The listing builds one solid part. Answer for the finished solid, in the listing's coordinates (mm). A direction names the side the tool comes from. Coordinates: 2 decimals unless noted, no trailing zeros. Write each loop counter-clockwise with the first axis right and the second up, starting at its lowest first coordinate (ties: lowest second). Pieces come first, ordered by that corner, then holes.
Autodesk Inventor part; units mm, degrees
ref_plane "YZ Plane" through (0, 0, 0) normal (1, 0, 0) x (0, 1, 0)
ref_plane "XZ Plane" through (0, 0, 0) normal (0, 1, 0) x (-1, 0, 0)
ref_plane "XY Plane" through (0, 0, 0) normal (0, 0, 1) x (1, 0, 0)
sketch "Sketch1" plane through (0, 0, 0) normal (0, 1, 0) x (-1, 0, 0)
  line L0 (0, 0) -> (8.89, 0)
  line L1 (8.89, 0) -> (8.89, -16.002)
  line L2 (8.89, -16.002) -> (0, -16.002)
  line L3 (0, -16.002) -> (0, 0)
  dimension "d0" = 8.89
  dimension "d1" = 16.002
extrude "Extrusion1" add sketch "Sketch1" along normal blind 2.54
sketch "Sketch5" plane through (0, 2.54, 0) normal (0, 1, 0) x (1, 0, 0)
  line L0 (-8.89, 0) -> (0, 0)
  line L1 (0, 0) -> (0, 16.002)
  line L2 (0, 16.002) -> (-8.89, 16.002)
  line L3 (-8.89, 16.002) -> (-8.89, 0)
  line L4 (0, 0) -> (-8.89, 0)
  line L5 (-5.7785, 0) -> (-6.6294, 0.9271)
  line L6 (-6.6294, 0.9271) -> (-6.6294, 1.6764)
  line L7 (-6.6294, 1.6764) -> (-2.2606, 1.6764)
  line L8 (-2.2606, 1.6764) -> (-2.2606, 0.9271)
  line L9 (-2.2606, 0.9271) -> (-3.1115, 0)
  line L10 (-8.89, 0) -> (-8.89, 16.002)
  line L11 (-8.89, 3.81) -> (0, 3.81)
  point P0 (-4.445, 1.6764)
  point P1 (-4.445, 3.81)
  dimension "d19" = 2.667
  dimension "d20" = 4.3688
  dimension "d21" = 0.9271
  dimension "d23" = 1.6764
  dimension "d24" = 3.81
extrude "Extrusion4" add sketch "Sketch5" along normal blind 3.175 contours L3 L11 L1 L0 L9 L8 L7 L6 L5
sketch "Sketch6" plane through (0, 2.54, 0) normal (0, 1, 0) x (1, 0, 0)
  line L0 (-3.1115, 0) -> (-2.2606, 0.9271)
  line L1 (-2.2606, 0.9271) -> (-2.2606, 1.6764)
  line L2 (-2.2606, 1.6764) -> (-6.6294, 1.6764)
  line L3 (-6.6294, 1.6764) -> (-6.6294, 0.9271)
  line L4 (-6.6294, 0.9271) -> (-5.7785, 0)
  line L5 (-5.7785, 0) -> (-3.1115, 0)
  point P0 (0, 0)
extrude "Extrusion5" cut sketch "Sketch6" against normal blind 1.016
fillet "Fillet3" radius 1.27 6 edges at (-8.89, 1.27, -16.002) (0, 1.27, -16.002) (-8.89, 2.8575, 0) (-8.89, 4.1275, -3.81) (0, 4.1275, -3.81) (0, 2.8575, 0)
sketch "Sketch8" plane through (0, 2.54, 0) normal (0, 1, 0) x (1, 0, 0)
  line L0 (-7.62, 16.002) -> (-1.27, 16.002)
  line L1 (-6.1595, 16.002) -> (-6.1595, 11.557)
  line L2 (-2.7305, 16.002) -> (-2.7305, 11.557)
  arc A0 (-6.1595, 11.557) -> (-2.7305, 11.557) centre (-4.445, 11.557) ccw
  point P0 (0, 0)
  point P1 (-4.445, 16.002)
  dimension "d37" = 3.429
  dimension "d38" = 4.445
extrude "Extrusion7" cut sketch "Sketch8" against normal blind 25.4
fillet "Fillet4" radius 1.016 2 edges at (-2.7305, 1.27, -16.002) (-6.1595, 1.27, -16.002)
properties part number "HallEffectSpoolSensorMount2" material "ABS Plastic"
Q1. Given pin 1 (2 mm diameter, centred on x = -5, y = 3.5, fed in from +Z); pin 2 (0.8 mm diameter, centred on x = -5, z = -0.5, fed in from +Y); pin 3 (4.5 mm diameter, centred on x = -4, z = -8, fed in from +Y), each flat-ended and moving along its own axis, determine where each tip first touches the part or whether it passes through.
Answers below:
pin 1: stops at z = 0
pin 2: stops at y = 1.52
pin 3: stops at y = 2.54
Q2. The part is cut by section B-B, the plane y = 0.85. Write down the section's boundary in (x, z) (1 decimal).
Answers below:
outline: (-8.9, -14.7) arc R1.3 ccw to (-7.6, -16) - (-7.2, -16) arc R1 ccw to (-6.2, -15) - (-6.2, -11.6) arc R1.7 cw to (-2.7, -11.6) - (-2.7, -15) arc R1 ccw to (-1.7, -16) - (-1.3, -16) arc R1.3 ccw to (0, -14.7) - (0, -1.3) arc R1.3 ccw to (-1.3, 0) - (-7.6, 0) arc R1.3 ccw to (-8.9, -1.3) - close
Q3. The part is cut by section A-A, the plane z = -13.5. Write down the section's boundary in (x, y).
Answers below:
outline: (-8.89, 0) - (-6.16, 0) - (-6.16, 2.54) - (-8.89, 2.54) - close; (-2.73, 0) - (0, 0) - (0, 2.54) - (-2.73, 2.54) - close
Q4. Find the intervals of material crossed by probe 1 along Y at (x, z) = (-3.5, -4); probe 2 along Z at (x, y) = (-5.5, 2.65); probe 3 along Z at (x, y) = (-6, 4.95), in increasing order.
Answers below:
probe 1: y = 0 to 2.54
probe 2: z = -3.81 to -1.68
probe 3: z = -3.81 to -1.68, -0.24 to 0
Q5. Which of the six approach directions +Z, -Z, +X, -X, +Y, -Y give full straight-line access (tool end or side, diameter ignored) to faces 1 (the face through (-8.508, 4.15, -3.448)), 2 (the face through (-4, 1.524, -1)), 3 (the face through (-4, 4, -3.81)), 4 (the face through (-6.465, 1.252, -15.712))?
Answers below:
face 1: -Z, -X, +Y
face 2: +Y
face 3: -Z, +X, -X, +Y
face 4: -Z, +Y, -Y
Q6. The part is cut by section C-C, the plane x = -8. Write down the section's boundary in (y, z) (3 decimals).
Answers below:
outline: (0, -15.944) - (2.54, -15.944) - (2.54, -3.752) - (5.715, -3.752) - (5.715, -0.058) - (0, -0.058) - close
Q7. Determine the mould class of faces 5 (the face through (-4, 4, -1.676)), 6 (the face through (-0.36, 1.29, -15.62)), 7 (the face through (-4, 2.54, -9)) for opening direction X: released by +X, released by -X, zero draft, split by the parting line, or undercut.
Answers below:
face 5: undercut
face 6: released by +X
face 7: zero draft
Q8. The part is cut by section D-D, the plane z = -11. Write down the section's boundary in (x, y), then the cut area to 3 significant figures.
Answers below:
outline: (-8.89, 0) - (-6.07, 0) - (-6.07, 2.54) - (-8.89, 2.54) - close; (-2.82, 0) - (0, 0) - (0, 2.54) - (-2.82, 2.54) - close
area: 14.3 mm2
